Model file for the job. Use its own axes, mm. A direction names the side the tool comes from. Coordinates: 2 decimals unless noted, no trailing zeros. Order: outer loops, then holes, each group sorted by start corner. A loop starts at its lowest first (then second) coordinate and runs counter-clockwise, first axis right, second up. Notation, with made-up numbers: (-5, -7.75) -> (32, -7.75) arc R21 cw to (32, 0.25) -> close; hole circle Ø9 at (85, -37). An arc over 180 degrees is marked (long way). Return JSON: item names as keys, results as strings. Group by question number.
1) Probe line 1 (Z direction, x = 0, y = 11.5); line 2 (X direction, y = 14, z = 2.25). List the from-to ranges inside material, lowest first.
2) Cut at B-B (y = 25.5). Write the cut outline in (x, z).
3) Pull direction X, two halves, no side cores. Call faces 1 (the cylindrical face through (3.2, 9.1, -2.4)), 2 (the flat face through (-3.912, 32.112, -2.224)), 3 (the cylindrical face through (-2.307, 29.867, -4.436)): +X half, -X half, draft (parallel to the pull), parting line (faces both ways), or undercut.
4) Which spindle directions (+Z, -Z, +X, -X, +Y, -Y) get a long thin tool onto all of the face, cutting with end or side? Do faces 4 (the flat face through (-4, 20, 4)), 5 (the flat face through (0, 32, 4.5)), 6 (the flat face through (4.1, 24, -2.4)). Say none if no direction does.
5) Flat gauge pins, fed straight in: pin 1 (5 mm diameter, centred on x = 0, z = 0, fed in from -Y); pin 2 (1 mm diameter, centred on x = 1, y = 33, fed in from -Z); pin 3 (1 mm diameter, centred on x = -3, y = 18.5, fed in from +Z); pin 4 (2.5 mm diameter, centred on y = 10, z = 0, fed in from -X). Where does each tip first touch, or does it go through?
6) Cut at C-C (z = 1.25). State how many separate pieces and enclosed holes the cut face has, and give its area (3 significant figures).
7) Cut at A-A (y = 11). Write the cut outline in (x, z).
from build123d import *

# Parameters (mm, degrees)
F0_R            = 8
F1_DEPTH        = 20
F2_R            = 5
F3_DEPTH        = 20
F5_DEPTH        = 16
F5_COPIES_COUNT = 3
F6_SIZE         = 0.49999
F7_R            = 0.5
F9_D            = 8
F9_DEPTH        = 18
F9_TIP          = 2.4034424761
F10_R           = 2.1
F11_DEPTH       = 8.25
F12_SIZE        = 3


# Not quite as in the source:
# - a fillet or chamfer is up to 0.001 mm smaller than in the source, because OpenCascade refuses the exact size
# - a pattern or mirror of a feature is missing from the dataset's text; its kind, count and spacing are read off the source's solid


with BuildPart() as f1:
    # F0 (on Front) → F1 (new body)
    with BuildSketch(Plane.XZ):
        Circle(F0_R)
    extrude(amount=-F1_DEPTH)

    # F2 (on face) → F3 (join)
    with BuildSketch(Plane(origin=(0, 20, 0), x_dir=(-1, 0, 0), z_dir=(0, 1, 0))):
        Circle(F2_R)
    extrude(amount=F3_DEPTH)

    # F4 (on face) → F5 (cut)
    with BuildSketch(Plane(origin=(0, 40, 0), x_dir=(-1, 0, 0), z_dir=(0, 1, 0))):
        with BuildLine():
            ThreePointArc((2.1794494718, 4.5), (0, 5), (-2.1794494718, 4.5))
            Line((-2.1794494718, 4.5), (2.1794494718, 4.5))
        make_face()
    f5 = extrude(amount=-F5_DEPTH, mode=Mode.SUBTRACT)

    # F5_copies: F5 ×3 about axis
    f5_copies_axis = Axis((0, 0, 0), (0, 1, 0))
    for i in range(1, F5_COPIES_COUNT):
        add(f5.rotate(f5_copies_axis, i * 360 / F5_COPIES_COUNT), mode=Mode.SUBTRACT)

    # F6 (size 0.5 in the source; OpenCascade refuses exactly that, so slightly less here)
    f6_edges = [f1.edges().sort_by_distance(p)[0] for p in [
        (4.330127, 40, 2.5),
        (-4.996709, 40, -0.18139),
        (0, 40, -5),
        (-4.236582, 40, 2.655443),
    ]]
    chamfer(f6_edges, length=F6_SIZE)

    # F7
    f7_edges = [f1.edges().sort_by_distance(p)[0] for p in [
        (-8, 20, 0),
        (5, 20, 0),
    ]]
    fillet(f7_edges, radius=F7_R)

    # F9
    with Locations(Plane.XZ):
        with Locations((0, 0)):
            Hole(F9_D / 2, depth=F9_DEPTH)
            with Locations((0, 0, -(F9_DEPTH + F9_TIP / 2))):  # 118° drill point
                Cone(0, F9_D / 2, F9_TIP, mode=Mode.SUBTRACT)

    # F10 (on Right) → F11 (cut, symmetric)
    with BuildSketch(Plane.YZ):
        with Locations((10, 0)):
            Circle(F10_R)
    extrude(amount=F11_DEPTH, both=True, mode=Mode.SUBTRACT)

    # F12
    f12_edges = [f1.edges().sort_by_distance(p)[0] for p in [
        (-8, 0, 0),
    ]]
    chamfer(f12_edges, length=F12_SIZE)


solid = f1.part
Answers below:
{
 "1": {"line 1": "z = -8 to -4, 4 to 8", "line 2": "x = -7.68 to -3.31, 3.31 to 7.68"},
 "2": {"outline": "(-4.99, -0.36) -> (-2.81, -4.14) arc R5 ccw to (2.81, -4.14) -> (4.99, -0.36) arc R5 ccw to (2.18, 4.5) -> (-2.18, 4.5) arc R5 ccw to start"},
 "3": {"face 1": "undercut", "face 2": "-X half", "face 3": "parting line"},
 "4": {"face 4": "+Y", "face 5": "+Z, +X, -X, +Y", "face 6": "-Z, +X, +Y"},
 "5": {"pin 1": "stops at y = 18.9", "pin 2": "stops at z = -4.97", "pin 3": "stops at z = 7.6", "pin 4": "passes through"},
 "6": {"separate pieces": "3", "enclosed holes": "0", "area": "328 mm^2"},
 "7": {"outline": "(-7.78, -1.85) arc R8 ccw to (7.78, -1.85) -> (3.55, -1.85) arc R4 cw to (-3.55, -1.85) -> close; (-7.78, 1.85) -> (-3.55, 1.85) arc R4 cw to (3.55, 1.85) -> (7.78, 1.85) arc R8 ccw to start"}
}
